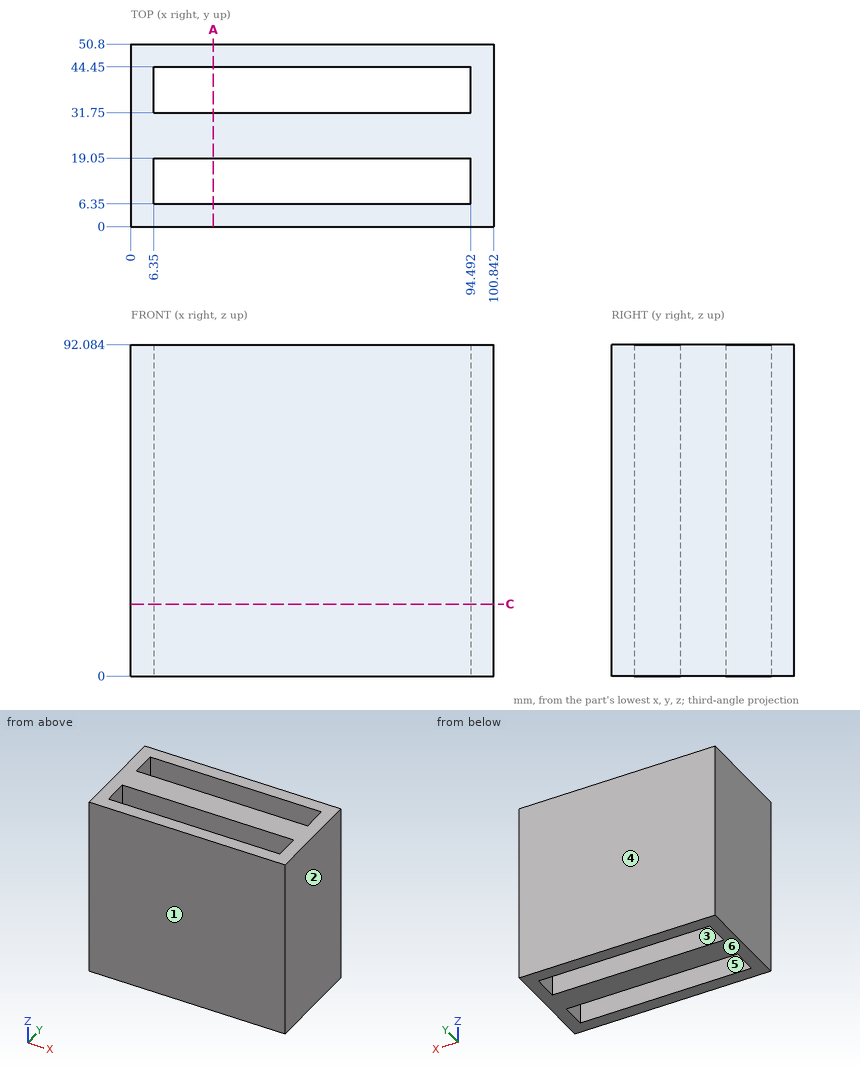
Can you work these out from the drawing? Everything is in mm from the part's minimum corner. A direction names the side the tool comes from. Coordinates: 2 decimals unless noted, no trailing zeros. Loops run counter-clockwise (first coordinate to the right, second up) from the corner with the lowest first, then second, coordinate; pieces in that order, holes last. Notation, with made-up numbers: M -4,0 L 40,0 A8 cw 40,15 Z; hole C -20.75,52 d9. An arc over 180 degrees is marked long. One line per item, written item: value.
1. Please list where these lines run through material, in increasing order: probe 1 along Y at (x, z) = (80, 66); probe 2 along X at (y, z) = (17.5, 45.5).
Geometry says:
probe 1: y = 0 to 6.35, 19.05 to 31.75, 44.45 to 50.8
probe 2: x = 0 to 6.35, 94.49 to 100.84
2. Thinking about a two-plate mould opening in Y: for the marked faces 1, 2, 3 and 4, which applies, +Y half, -Y half, draft (parallel to the pull), parting line (faces both ways), or undercut?
Geometry says:
face 1: -Y half
face 2: draft
face 3: undercut
face 4: +Y half
3. Imagine slicing it at C-C (z = 20). List the corners of the cut face in (x, y) for me.
Geometry says:
outline: M 0,0 L 100.84,0 L 100.84,50.8 L 0,50.8 Z; hole M 6.35,6.35 L 94.49,6.35 L 94.49,19.05 L 6.35,19.05 Z; hole M 6.35,31.75 L 94.49,31.75 L 94.49,44.45 L 6.35,44.45 Z
4. Will this pin go through, and if not, where does the flat tip stop? pin 1 Ø6.5 at (y, z) = (36, 58.5) entering from -X.
Geometry says:
pin 1: stops at x = 0
5. On a 3-axis mill with a long thin cutter (end or side, diameter ignored), from which of +Z, -Z, +X, -X, +Y, -Y can I reach the whole of each face in a straight line? I mean the marked faces 5 and 6. Say none if no direction works.
Geometry says:
face 5: +Z, -Z
face 6: -Z, +X, -X, +Y, -Y
6. Imagine slicing it at A-A (x = 23). State how many separate pieces and enclosed holes the cut face has, and give its area (3 significant figures).
Geometry says:
separate pieces: 3
enclosed holes: 0
area: 2,340 mm2
